from build123d import *

# Parameters (mm, degrees)
BOSS_EXTRUDE1_DEPTH = 179.4
FILLET3_R           = 10
CUT_EXTRUDE3_REACH  = 193.526
SKETCH4_R           = 1.55
CUT_EXTRUDE5_REACH  = 192.528
SKETCH7_W           = 26
SKETCH7_H           = 20
SKETCH7_W_2         = 25.4
SKETCH7_W_3         = 2
FILLET6_R           = 2
FILLET7_R           = 2


with BuildPart() as part:
    # Sketch1 → Boss-Extrude1 (new body)
    with BuildSketch(Plane(origin=(0, 0, 0), x_dir=(0, 0, -1), z_dir=(1, 0, 0))):
        Polygon((-2.5, -15.488635846), (-2.5, -31.932011519), (45.315389352, -51.619548933), (2.5, -29.045260173), (2.5, -15.488635846), align=None)
    extrude(amount=BOSS_EXTRUDE1_DEPTH)

    # Fillet3
    fillet3_edges = [part.edges().sort_by_distance(p)[0] for p in [
        (89.7, -29.045260173, -2.5),
        (89.7, -31.932011519, 2.5),
    ]]
    fillet(fillet3_edges, radius=FILLET3_R)

    # Sketch4 → Cut-Extrude3 (cut, up to next)
    with BuildSketch(Plane(origin=(0, 0, -2.5), x_dir=(-1, 0, 0), z_dir=(0, 0, -1)), mode=Mode.PRIVATE) as cut_extrude3_sk1:
        with Locations(Location((-171.9, -20.488635846, 0), (0, 0, 90))):
            Circle(SKETCH4_R)
    cut_extrude3_tool1 = extrude(cut_extrude3_sk1.sketch, amount=-CUT_EXTRUDE3_REACH, mode=Mode.PRIVATE) & part.part
    # Sketch4 → Cut-Extrude3 (cut, up to next)
    with BuildSketch(Plane(origin=(0, 0, -2.5), x_dir=(-1, 0, 0), z_dir=(0, 0, -1)), mode=Mode.PRIVATE) as cut_extrude3_sk2:
        with Locations(Location((-7.5, -20.488635846, 0), (0, 0, 90))):
            Circle(SKETCH4_R)
    cut_extrude3_tool2 = extrude(cut_extrude3_sk2.sketch, amount=-CUT_EXTRUDE3_REACH, mode=Mode.PRIVATE) & part.part
    # Sketch4 → Cut-Extrude3 (cut, up to next)
    with BuildSketch(Plane(origin=(0, 0, -2.5), x_dir=(-1, 0, 0), z_dir=(0, 0, -1)), mode=Mode.PRIVATE) as cut_extrude3_sk3:
        with Locations(Location((-89.7, -20.488635846, 0), (0, 0, 90))):
            Circle(SKETCH4_R)
    cut_extrude3_tool3 = extrude(cut_extrude3_sk3.sketch, amount=-CUT_EXTRUDE3_REACH, mode=Mode.PRIVATE) & part.part
    add(cut_extrude3_tool1.solids().sort_by_distance((171.9, -20.488636, -2.5))[0], mode=Mode.SUBTRACT)
    add(cut_extrude3_tool2.solids().sort_by_distance((7.5, -20.488636, -2.5))[0], mode=Mode.SUBTRACT)
    add(cut_extrude3_tool3.solids().sort_by_distance((89.7, -20.488636, -2.5))[0], mode=Mode.SUBTRACT)

    # Sketch7 → Cut-Extrude5 (cut, up to next)
    with BuildSketch(Plane(origin=(0, -21.695908288, 11.439104164), x_dir=(1, 0, 0), z_dir=(0, 0.8845784624906722, -0.466391406114691)), mode=Mode.PRIVATE) as cut_extrude5_sk1:
        with Locations((144.4, 54.15993145)):
            Rectangle(SKETCH7_W, SKETCH7_H)
    cut_extrude5_tool1 = extrude(cut_extrude5_sk1.sketch, amount=-CUT_EXTRUDE5_REACH, mode=Mode.PRIVATE) & part.part
    # Sketch7 → Cut-Extrude5 (cut, up to next)
    with BuildSketch(Plane(origin=(0, -21.695908288, 11.439104164), x_dir=(1, 0, 0), z_dir=(0, 0.8845784624906722, -0.466391406114691)), mode=Mode.PRIVATE) as cut_extrude5_sk2:
        with Locations((100.4, 54.15993145)):
            Rectangle(SKETCH7_W, SKETCH7_H)
    cut_extrude5_tool2 = extrude(cut_extrude5_sk2.sketch, amount=-CUT_EXTRUDE5_REACH, mode=Mode.PRIVATE) & part.part
    # Sketch7 → Cut-Extrude5 (cut, up to next)
    with BuildSketch(Plane(origin=(0, -21.695908288, 11.439104164), x_dir=(1, 0, 0), z_dir=(0, 0.8845784624906722, -0.466391406114691)), mode=Mode.PRIVATE) as cut_extrude5_sk3:
        with Locations((56.4, 54.15993145)):
            Rectangle(SKETCH7_W, SKETCH7_H)
    cut_extrude5_tool3 = extrude(cut_extrude5_sk3.sketch, amount=-CUT_EXTRUDE5_REACH, mode=Mode.PRIVATE) & part.part
    # Sketch7 → Cut-Extrude5 (cut, up to next)
    with BuildSketch(Plane(origin=(0, -21.695908288, 11.439104164), x_dir=(1, 0, 0), z_dir=(0, 0.8845784624906722, -0.466391406114691)), mode=Mode.PRIVATE) as cut_extrude5_sk4:
        with Locations((12.7, 54.15993145)):
            Rectangle(SKETCH7_W_2, SKETCH7_H)
    cut_extrude5_tool4 = extrude(cut_extrude5_sk4.sketch, amount=-CUT_EXTRUDE5_REACH, mode=Mode.PRIVATE) & part.part
    # Sketch7 → Cut-Extrude5 (cut, up to next)
    with BuildSketch(Plane(origin=(0, -21.695908288, 11.439104164), x_dir=(1, 0, 0), z_dir=(0, 0.8845784624906722, -0.466391406114691)), mode=Mode.PRIVATE) as cut_extrude5_sk5:
        with Locations((178.4, 54.15993145)):
            Rectangle(SKETCH7_W_3, SKETCH7_H)
    cut_extrude5_tool5 = extrude(cut_extrude5_sk5.sketch, amount=-CUT_EXTRUDE5_REACH, mode=Mode.PRIVATE) & part.part
    add(cut_extrude5_tool1.solids().sort_by_distance((144.4, -46.955635, -36.469605))[0], mode=Mode.SUBTRACT)
    add(cut_extrude5_tool2.solids().sort_by_distance((100.4, -46.955635, -36.469605))[0], mode=Mode.SUBTRACT)
    add(cut_extrude5_tool3.solids().sort_by_distance((56.4, -46.955635, -36.469605))[0], mode=Mode.SUBTRACT)
    add(cut_extrude5_tool4.solids().sort_by_distance((12.7, -46.955635, -36.469605))[0], mode=Mode.SUBTRACT)
    add(cut_extrude5_tool5.solids().sort_by_distance((178.4, -46.955635, -36.469605))[0], mode=Mode.SUBTRACT)

    # Fillet6
    fillet6_edges = [part.edges().sort_by_distance(p)[0] for p in [
        (25.4, -43.131220066, -27.181196576),
        (69.4, -43.131220066, -27.181196576),
        (43.4, -43.131220066, -27.181196576),
        (113.4, -43.131220066, -27.181196576),
        (87.4, -43.131220066, -27.181196576),
        (177.4, -43.131220066, -27.181196576),
        (157.4, -43.131220066, -27.181196576),
        (131.4, -43.131220066, -27.181196576),
    ]]
    fillet(fillet6_edges, radius=FILLET6_R - 0.0001)  # a hair under: the kernel refuses the full size

    # Fillet7
    fillet7_edges = [part.edges().sort_by_distance(p)[0] for p in [
        (89.7, -15.488635846, 2.5),
    ]]
    fillet(fillet7_edges, radius=FILLET7_R)


solid = part.part
Check sheet for the modelled part. Datum: model origin and axes. Units: mm. A direction names the side the tool comes from. Round coordinates to 2 decimals unless told otherwise and drop trailing zeros. Loops run counter-clockwise (first coordinate to the right, second up) from the corner with the lowest first, then second, coordinate; pieces in that order, holes last. Notation, with made-up numbers: M -24.75,63 L -3.75,63 A24 ccw -3.75,79 Z; hole C 83,64 d8. An arc over 180 degrees is marked long. One line per question, with ' | ' between items. Start each with the question number.
Item 1: Scan lines: probe 1 along Z at (x, y) = (142.5, -23.5); probe 2 along Y at (x, z) = (171, 1); probe 3 along Y at (x, z) = (89.7, -1.45). Record each from-to range of solid material in increasing order.
Item 2: Section check A-A (x = 7.5). Record the boundary of the cut face in (y, z).
Item 3: Release check for a two-part mould opening along X. For faces 1 (the face through (131.4, -47, -35)), 2 (the face through (88.187, -20.825, -0.035)), 3 (the face through (0, -31, -6)), 4 (the face through (88.44, -39.68, -22.67)) record: released by +X, released by -X, zero draft, split by the parting line, or undercut.
Item 4: Set-up check for faces 5 (the face through (179.4, -31, -6)), 6 (the face through (88, -19, -2.5)): record each of +Z, -Z, +X, -X, +Y, -Y from which the full face is reachable in a straight line by a thin tool's end or side.
Item 5: Gauge pin test, flat ends, axial feed: pin 1 Ø2.5 at (y, z) = (-49, -38) entering from -X; pin 2 Ø12 at (x, z) = (146.5, -35) entering from -Y; pin 3 Ø5 at (x, y) = (171.9, -20.49) entering from -Z; pin 4 Ø2.5 at (y, z) = (-46.5, -33) entering from +X. Record the tip position at first contact, or that the pin passes through.
Item 6: Section check C-C (y = -49). Record the boundary of the cut face in (x, z), and give its area (3 significant figures).
Item 7: Section check B-B (x = 39.5). Record the boundary of the cut face in (y, z).
Item 8: Section check D-D (x = 171.9). Record the boundary of the cut face in (y, z), and give its area (3 significant figures).
Worked out:
1) probe 1: -2.51 to 2.5 | probe 2: -30.5 to -21.75, -19.23 to -15.55 | probe 3: -33.2 to -22.04, -18.94 to -15.49
2) outline: M -43.97,-26.74 L -42.29,-27.62 L -31.86,-7.84 A10 cw -23.01,-2.5 L -22.04,-2.5 L -22.04,2.5 L -25.23,2.5 A10 ccw -34.48,-3.69 Z; M -18.94,-2.5 L -15.49,-2.5 L -15.49,0.5 A2 ccw -17.49,2.5 L -18.94,2.5 Z
3) face 1: undercut | face 2: undercut | face 3: released by -X | face 4: zero draft
4) face 5: +Z, -Z, +X, +Y, -Y | face 6: -Z, +X, -X, +Y
5) pin 1: x = 25.4 | pin 2: through | pin 3: z = -2.5 | pin 4: x = 177.4
6) outline: M 25.4,-40.35 L 43.4,-40.35 L 43.4,-38.95 L 25.4,-38.95 Z; M 69.4,-40.35 L 87.4,-40.35 L 87.4,-38.95 L 69.4,-38.95 Z; M 113.4,-40.35 L 131.4,-40.35 L 131.4,-38.95 L 113.4,-38.95 Z; M 157.4,-40.35 L 177.4,-40.35 L 177.4,-38.95 L 157.4,-38.95 Z | area: 103 mm^2
7) outline: M -51.62,-45.32 L -31.86,-7.84 A10 cw -23.01,-2.5 L -15.49,-2.5 L -15.49,0.5 A2 ccw -17.49,2.5 L -25.23,2.5 A10 ccw -34.48,-3.69 Z
8) outline: M -51.62,-45.32 L -31.86,-7.84 A10 cw -23.01,-2.5 L -22.04,-2.5 L -22.04,2.5 L -25.23,2.5 A10 ccw -34.48,-3.69 Z; M -18.94,-2.5 L -15.49,-2.5 L -15.49,0.5 A2 ccw -17.49,2.5 L -18.94,2.5 Z | area: 175 mm^2
